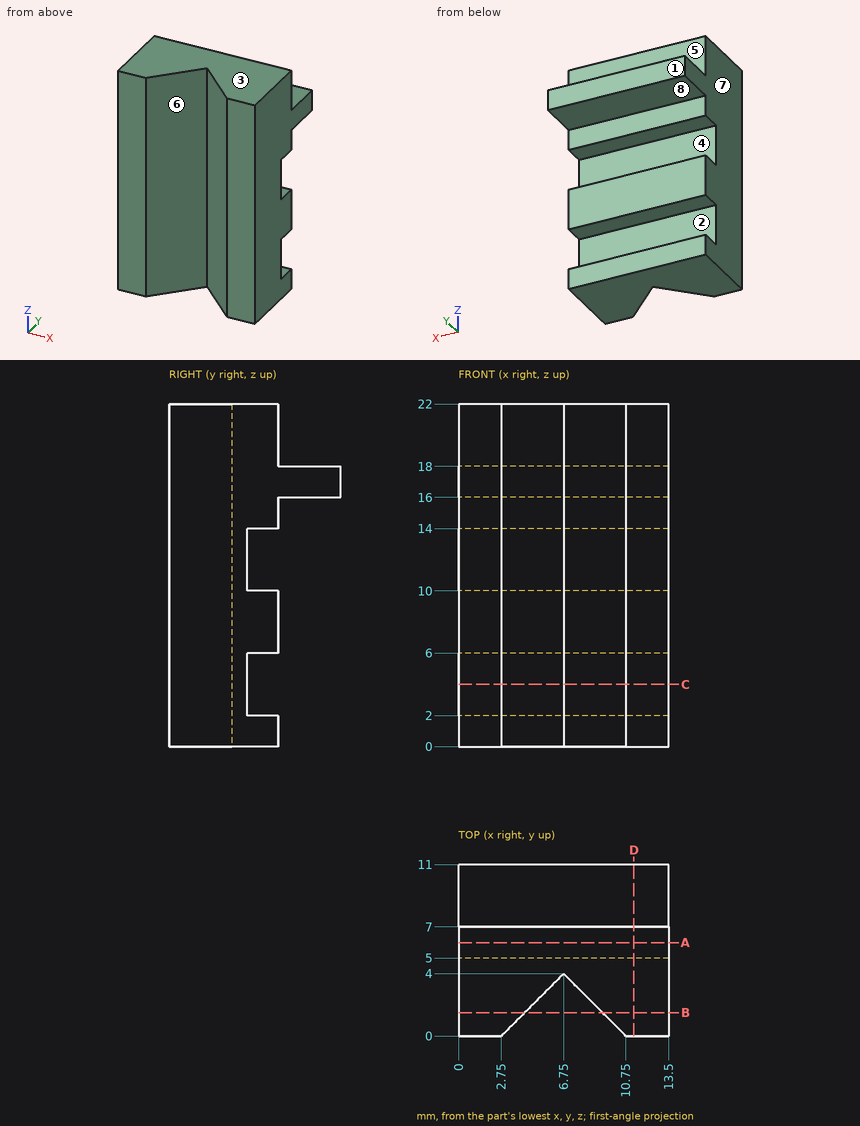
Job drawing, mm, ordinate dimensions from the low corner. One solid piece. A direction names the side the tool comes from. Give positions to 0.01 mm unless a question says otherwise; leave off trailing zeros. Write each loop counter-clockwise with the first axis right and the second up, starting at its lowest first coordinate (ties: lowest second). Pieces come first, ordered by that corner, then holes. Notation, with made-up numbers: (5, -33.5) -> (51, -33.5) arc R20 ccw to (51, -20.5) -> close; hole circle Ø2 at (13, 78). An arc over 180 degrees is marked (long way). Return JSON: item names as keys, results as strings.
Item 1: Drill centre lines: probe 1 along Z at (x, y) = (11.75, 6.25); probe 2 along Y at (x, z) = (2, 12.75); probe 3 along X at (y, z) = (3, 4.5). Where is each one in solid material? Low to high.
Answer below:
{"probe 1": "z = 0 to 2, 6 to 10, 14 to 22", "probe 2": "y = 0 to 5", "probe 3": "x = 0 to 5.75, 7.75 to 13.5"}
Item 2: Band-saw the part on A-A (y = 6). List the corners of the cut face in (x, z), then the cut area to 3 significant figures.
Answer below:
{"outline": "(0, 0) -> (13.5, 0) -> (13.5, 2) -> (0, 2) -> close; (0, 6) -> (13.5, 6) -> (13.5, 10) -> (0, 10) -> close; (0, 14) -> (13.5, 14) -> (13.5, 22) -> (0, 22) -> close", "area": "189 mm2"}
Item 3: Band-saw the part on C-C (z = 4). List the corners of the cut face in (x, y), then the cut area to 3 significant figures.
Answer below:
{"outline": "(0, 0) -> (2.75, 0) -> (6.75, 4) -> (10.75, 0) -> (13.5, 0) -> (13.5, 5) -> (0, 5) -> close", "area": "51.5 mm2"}
Item 4: Band-saw the part on D-D (x = 11.25). List the corners of the cut face in (y, z).
Answer below:
{"outline": "(0, 0) -> (7, 0) -> (7, 2) -> (5, 2) -> (5, 6) -> (7, 6) -> (7, 10) -> (5, 10) -> (5, 14) -> (7, 14) -> (7, 16) -> (11, 16) -> (11, 18) -> (7, 18) -> (7, 22) -> (0, 22) -> close"}
Item 5: Band-saw the part on B-B (y = 1.5). List the corners of the cut face in (x, z).
Answer below:
{"outline": "(0, 0) -> (4.25, 0) -> (4.25, 22) -> (0, 22) -> close; (9.25, 0) -> (13.5, 0) -> (13.5, 22) -> (9.25, 22) -> close"}
Item 6: Drop flat-ended pins along their axis: pin 1 (4.5 mm diameter, centred on x = 4.5, z = 4.5, fed in from +Y); pin 2 (1.2 mm diameter, centred on x = 5.5, y = 8.5, fed in from +Z); pin 3 (1 mm diameter, centred on x = 6, y = 6.5, fed in from -Z); pin 4 (2 mm diameter, centred on x = 5.5, z = 12, fed in from +Y). Give the stop position or say it passes through.
Answer below:
{"pin 1": "stops at y = 7", "pin 2": "stops at z = 18", "pin 3": "stops at z = 0", "pin 4": "stops at y = 5"}
Item 7: Tool access for the marked faces 4, 5, 6, 7 and 8: list every direction of +Z, -Z, +X, -X, +Y, -Y with a clear straight run to the whole face (end or side of a thin tool).
Answer below:
{"face 4": "+X, -X, +Y", "face 5": "+Z, +X, -X, +Y", "face 6": "+Z, -Z, -Y", "face 7": "+Z, -Z, -X, +Y, -Y", "face 8": "-Z, +X, -X, +Y"}
Item 8: Two-plate mould, pull along Z, no slides. Class the marked faces 1, 2 and 3: +Z half, -Z half, draft (parallel to the pull), parting line (faces both ways), or undercut.
Answer below:
{"face 1": "draft", "face 2": "undercut", "face 3": "+Z half"}
